The model under review builds one solid part; all positions refer to its coordinate system, in mm. Give positions to 0.01 mm unless a question says otherwise; leave off trailing zeros. Write each loop counter-clockwise with the first axis right and the second up, starting at its lowest first coordinate (ties: lowest second). Pieces come first, ordered by that corner, then holes.
from build123d import *

# Parameters (mm, degrees)
F0_R          = 22.5
F1_DEPTH      = 101.6
F3_DEPTH      = 22.501
F3_DEPTH_BACK = 22.501
F4_DEPTH      = 22.501
F4_DEPTH_BACK = 22.501
F6_DEPTH      = 83.079608795
F7_R          = 2.38125
F8_DEPTH      = 83.079608795
F9_R          = 2.38125
F9_R_2        = 6.985
F10_DEPTH     = 83.079608795


with BuildPart() as f1:
    # F0 (on Front) → F1 (new body)
    with BuildSketch(Plane.XZ):
        Circle(F0_R)
    extrude(amount=F1_DEPTH)

    # F2 (on Right) → F3 (cut, two sides)
    with BuildSketch(Plane.YZ) as f3_sk:
        Polygon((-106.5287748777, -38.457716324), (-83.0848926463, -22.5044), (-18.8056646404, 22.5044), (-103.6715880036, 26.2515861541), align=None)
    extrude(amount=-F3_DEPTH, mode=Mode.SUBTRACT)
    extrude(f3_sk.sketch, amount=F3_DEPTH_BACK, mode=Mode.SUBTRACT)

    # F2 (on Right) → F4 (cut, two sides)
    with BuildSketch(Plane.YZ) as f4_sk:
        Polygon((-12.2079484916, 22.5), (-76.4808926463, -22.5044), (27.3525305092, -35.9458737075), (27.3525305092, 27.8113950044), align=None)
    extrude(amount=-F4_DEPTH, mode=Mode.SUBTRACT)
    extrude(f4_sk.sketch, amount=F4_DEPTH_BACK, mode=Mode.SUBTRACT)

    # F5 (on Front) → F6 (cut, through all)
    with BuildSketch(Plane.XZ):
        with BuildLine():
            ThreePointArc((8.9661090106, -12.3234122389), (9.901471319, -11.5852693417), (10.7763073453, -10.7763073453))
            Line((10.7763073453, -10.7763073453), (9.0925093226, -9.0925093226))
            ThreePointArc((9.0925093226, -9.0925093226), (8.3968775712, -10.6832186102), (8.9661090106, -12.3234122389))
        make_face()
        with BuildLine():
            ThreePointArc((10.7763073453, -10.7763073453), (11.5852693417, -9.901471319), (12.3234122389, -8.9661090106))
            ThreePointArc((12.3234122389, -8.9661090106), (10.6832186102, -8.3968775712), (9.0925093226, -9.0925093226))
            Line((9.0925093226, -9.0925093226), (10.7763073453, -10.7763073453))
        make_face()
        with BuildLine():
            Line((12.460105368, -12.460105368), (10.7763073453, -10.7763073453))
            ThreePointArc((10.7763073453, -10.7763073453), (9.901471319, -11.5852693417), (8.9661090106, -12.3234122389))
            ThreePointArc((8.9661090106, -12.3234122389), (10.6832186102, -13.1557371194), (12.460105368, -12.460105368))
        make_face()
        with BuildLine():
            ThreePointArc((15.0539648438, -2.3739718792), (15.1934200268, -1.190625), (15.24, 0))
            ThreePointArc((15.24, 0), (15.1934200268, 1.190625), (15.0539648438, 2.3739718792))
            ThreePointArc((15.0539648438, 2.3739718792), (12.85875, 0), (15.0539648438, -2.3739718792))
        make_face()
        with BuildLine():
            ThreePointArc((15.0539648438, 2.3739718792), (15.1934200268, 1.190625), (15.24, 0))
            ThreePointArc((15.24, 0), (15.1934200268, -1.190625), (15.0539648438, -2.3739718792))
            ThreePointArc((15.0539648438, -2.3739718792), (16.8566872528, -1.7483346045), (17.62125, 0))
            ThreePointArc((17.62125, 0), (16.8566872528, 1.7483346045), (15.0539648438, 2.3739718792))
        make_face()
        with BuildLine():
            ThreePointArc((-2.3739718792, 15.0539648438), (0, 15.24), (2.3739718792, 15.0539648438))
            ThreePointArc((2.3739718792, 15.0539648437), (2.3794297741, 15.1469112649), (2.38125, 15.24))
            ThreePointArc((2.38125, 15.24), (-0.0930887351, 17.6194297741), (-2.3739718792, 15.0539648438))
        make_face()
        with BuildLine():
            ThreePointArc((-2.3739718792, 15.0539648438), (0, 12.85875), (2.3739718792, 15.0539648437))
            ThreePointArc((2.3739718792, 15.0539648438), (0, 15.24), (-2.3739718792, 15.0539648438))
        make_face()
        with BuildLine():
            ThreePointArc((2.38125, -15.24), (2.3794297741, -15.1469112649), (2.3739718792, -15.0539648437))
            ThreePointArc((2.3739718792, -15.0539648438), (0, -15.24), (-2.3739718792, -15.0539648438))
            ThreePointArc((-2.3739718792, -15.0539648438), (-0.0930887351, -17.6194297741), (2.38125, -15.24))
        make_face()
        with BuildLine():
            ThreePointArc((-12.3234122389, 8.9661090106), (-10.6832186102, 8.3968775712), (-9.0925093226, 9.0925093226))
            Line((-9.0925093226, 9.0925093226), (-10.7763073453, 10.7763073453))
            ThreePointArc((-10.7763073453, 10.7763073453), (-11.5852693417, 9.901471319), (-12.3234122389, 8.9661090106))
        make_face()
        with BuildLine():
            ThreePointArc((-12.3234122389, 8.9661090106), (-11.5852693417, 9.901471319), (-10.7763073453, 10.7763073453))
            Line((-10.7763073453, 10.7763073453), (-12.460105368, 12.460105368))
            ThreePointArc((-12.460105368, 12.460105368), (-13.1557371194, 10.6832186102), (-12.3234122389, 8.9661090106))
        make_face()
        with BuildLine():
            ThreePointArc((-8.3950573453, -10.7763073453), (-8.5763192085, -9.865042422), (-9.0925093226, -9.0925093226))
            Line((-9.0925093226, -9.0925093226), (-10.7763073453, -10.7763073453))
            ThreePointArc((-10.7763073453, -10.7763073453), (-9.901471319, -11.5852693417), (-8.9661090106, -12.3234122389))
            ThreePointArc((-8.9661090106, -12.3234122389), (-8.5423773613, -11.6008729213), (-8.3950573453, -10.7763073453))
        make_face()
        with BuildLine():
            ThreePointArc((-15.24, 0), (-15.1934200268, 1.190625), (-15.0539648438, 2.3739718792))
            ThreePointArc((-15.0539648438, 2.3739718792), (-17.62125, 0), (-15.0539648438, -2.3739718792))
            ThreePointArc((-15.0539648438, -2.3739718792), (-15.1934200268, -1.190625), (-15.24, 0))
        make_face()
        with BuildLine():
            ThreePointArc((9.0925093226, 9.0925093226), (10.6832186102, 8.3968775712), (12.3234122389, 8.9661090106))
            ThreePointArc((12.3234122389, 8.9661090106), (11.5852693417, 9.901471319), (10.7763073453, 10.7763073453))
            Line((10.7763073453, 10.7763073453), (9.0925093226, 9.0925093226))
        make_face()
        with BuildLine():
            ThreePointArc((-15.0539648438, -2.3739718792), (-13.4916653955, -1.6166872528), (-12.85875, 0))
            Line((-12.85875, 0), (-15.24, 0))
            ThreePointArc((-15.24, 0), (-15.1934200268, -1.190625), (-15.0539648438, -2.3739718792))
        make_face()
        with BuildLine():
            Line((-15.24, 0), (-12.85875, 0))
            ThreePointArc((-12.85875, 0), (-13.4916653955, 1.6166872528), (-15.0539648438, 2.3739718792))
            ThreePointArc((-15.0539648438, 2.3739718792), (-15.1934200268, 1.190625), (-15.24, 0))
        make_face()
        with BuildLine():
            Line((-10.7763073453, 10.7763073453), (-9.0925093226, 9.0925093226))
            ThreePointArc((-9.0925093226, 9.0925093226), (-8.5763192085, 9.865042422), (-8.3950573453, 10.7763073453))
            ThreePointArc((-8.3950573453, 10.7763073453), (-8.5423773613, 11.6008729213), (-8.9661090106, 12.3234122389))
            ThreePointArc((-8.9661090106, 12.3234122389), (-9.901471319, 11.5852693417), (-10.7763073453, 10.7763073453))
        make_face()
        with BuildLine():
            Line((9.0925093226, 9.0925093226), (10.7763073453, 10.7763073453))
            ThreePointArc((10.7763073453, 10.7763073453), (9.901471319, 11.5852693417), (8.9661090106, 12.3234122389))
            ThreePointArc((8.9661090106, 12.3234122389), (8.3968775712, 10.6832186102), (9.0925093226, 9.0925093226))
        make_face()
        with BuildLine():
            ThreePointArc((-2.3739718792, -15.0539648438), (0, -15.24), (2.3739718792, -15.0539648438))
            ThreePointArc((2.3739718792, -15.0539648437), (0, -12.85875), (-2.3739718792, -15.0539648438))
        make_face()
    extrude(amount=F6_DEPTH, mode=Mode.SUBTRACT)

    # F7 (on Front) → F8 (cut, through all)
    with BuildSketch(Plane.XZ):
        with Locations((10.7763073453, 10.7763073453)):
            Circle(F7_R)
    extrude(amount=F8_DEPTH, mode=Mode.SUBTRACT)

    # F9 (on Front) → F10 (cut, through all)
    with BuildSketch(Plane.XZ):
        with Locations((10.7763073453, -10.7763073453)):
            Circle(F9_R)
        with Locations((-10.7763073453, -10.7763073453)):
            Circle(F9_R)
        with Locations((-10.7763073453, 10.7763073453)):
            Circle(F9_R)
        Circle(F9_R_2)
    extrude(amount=F10_DEPTH, mode=Mode.SUBTRACT)


solid = f1.part
1) The part is to be moulded in two halves that separate along X. For faces 1 (the cylindrical face through (6.95, -46.58, 0.71)), 2 (the flat face through (9.69, -51.4, -0.32)), 3 (the cylindrical face through (-22.5, -47.5, 0.3)), 4 (the cylindrical face through (-9.48, -62.94, -8.78)), say which applies: +X half, -X half, draft (parallel to the pull), parting line (faces both ways), or undercut.
2) Consider section C-C, the plane x = -10.5. Give the boundary of the cut face in (y, z), then the cut area to 3 significant figures.
3) To check wall thickness, follow probe 1 along Z at (x, y) = (17, -60.5); probe 2 along Y at (x, z) = (-16, 2.5); probe 3 along Y at (x, z) = (-11, 17). State the ranges of each line that lie inside material, in increasing order.
4) Consider section A-A, the plane z = 5.5. Give the boundary of the cut face in (x, y).
5) Consider section B-B, the plane x = 0. Give the boundary of the cut face in (y, z) (3 decimals).
6) Consider section D-D, the plane z = 10. Give the boundary of the cut face in (x, y).
7) Insertion check: pin 1 (1.5 mm diameter, centred on y = -66.5, z = -11, fed in from +X); pin 2 (8 mm diameter, centred on x = -14, z = -1, fed in from +Y); pin 3 (6 mm diameter, centred on y = -33.5, z = 8.5, fed in from -X); pin 4 (11 mm diameter, centred on x = 0, z = 0, fed in from -Y). Each pin has a flat end and moves straight along its axis. Give the tip position at first contact, or say it passes through.
Answer block:
1. face 1: undercut
1. face 2: draft
1. face 3: parting line
1. face 4: undercut
2. outline: (-79.37, -19.9) - (-72.76, -19.9) - (-63.11, -13.14) - (-69.71, -13.14) - close; (-62.96, -8.41) - (-56.35, -8.41) - (-32.33, 8.41) - (-38.93, 8.41) - close; (-32.18, 13.14) - (-25.57, 13.14) - (-15.92, 19.9) - (-22.53, 19.9) - close
2. area: 200 mm2
3. probe 1: z = -11.31 to -6.69
3. probe 2: y = -47.37 to -40.77
3. probe 3: y = -26.67 to -20.06
4. outline: (-21.82, -43.09) - (-4.31, -43.09) - (-4.31, -36.49) - (-21.82, -36.49) - close; (4.31, -43.09) - (21.82, -43.09) - (21.82, -36.49) - (4.31, -36.49) - close
5. outline: (-83.079, -22.5) - (-76.475, -22.5) - (-69.507, -17.621) - (-76.111, -17.621) - close; (-69.309, -12.859) - (-62.705, -12.859) - (-54.317, -6.985) - (-60.921, -6.985) - close; (-40.97, 6.985) - (-34.366, 6.985) - (-25.977, 12.859) - (-32.581, 12.859) - close; (-25.78, 17.621) - (-19.176, 17.621) - (-12.208, 22.5) - (-18.812, 22.5) - close
6. outline: (-20.16, -36.66) - (-13.03, -36.66) - (-13.03, -30.06) - (-20.16, -30.06) - close; (-8.53, -36.66) - (8.53, -36.66) - (8.53, -30.06) - (-8.53, -30.06) - close; (13.03, -36.66) - (20.16, -36.66) - (20.16, -30.06) - (13.03, -30.06) - close
7. pin 1: stops at x = 19.9
7. pin 2: stops at y = -40.06
7. pin 3: stops at x = -21.62
7. pin 4: passes through
